For this review, use the dimensioned drawing (mm, ordinates from the lowest corner) and the shaded views. Give positions to 0.01 mm unless a question says otherwise; leave off trailing zeros. Order: outer loops, then holes, each group sorted by start corner. A loop starts at its lowest first (then second) coordinate and runs counter-clockwise, first axis right, second up.
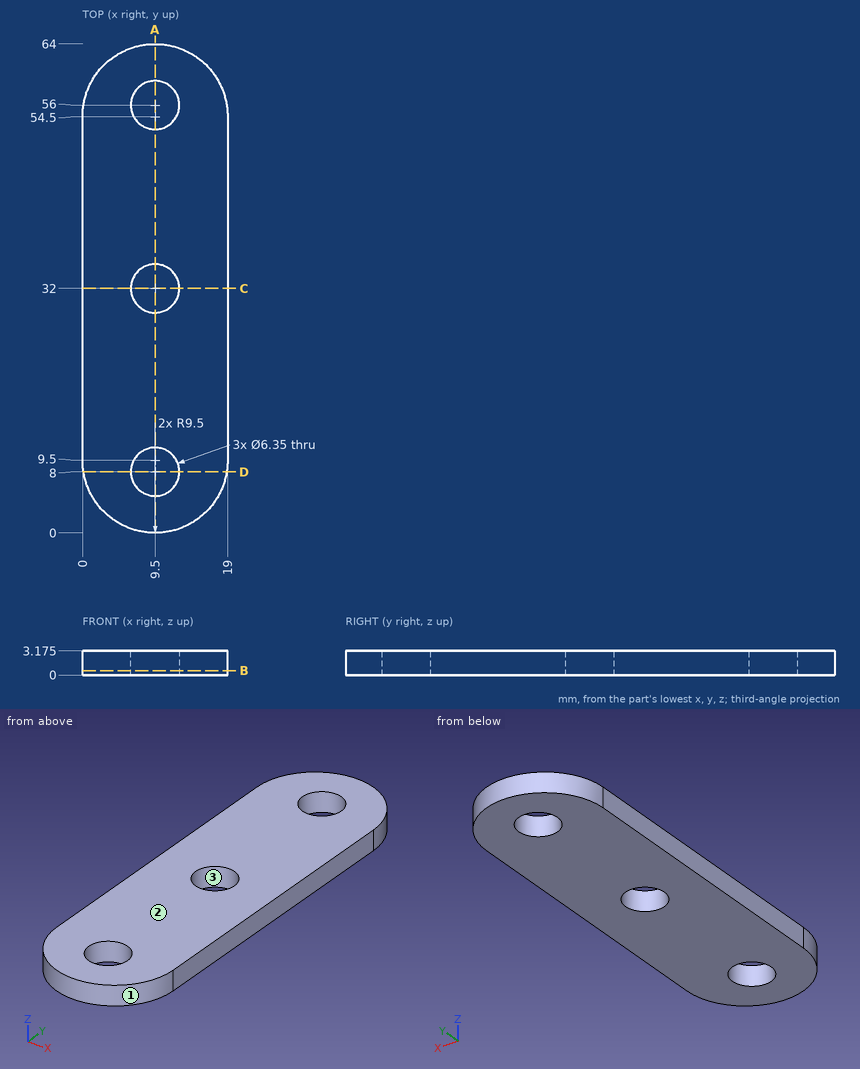
1. For pin 1 (5 mm diameter, centred on x = 9.5, y = 8, fed in from +Z), flat-tipped, find the tip position at first contact; note if it passes through.
Recorded:
pin 1: passes through
2. Draft analysis for pull direction X (two halves, no side actions). For the marked faces 1, 2 and 3, state which applies: pulls with the +X half, pulls with the -X half, needs draft (parallel to the pull), parting line crosses it, or undercut.
Recorded:
face 1: parting line crosses it
face 2: needs draft
face 3: undercut
3. For line 1 along Y through (x, z) = (9.5, 2) (3 decimals); line 2 along Y through (x, z) = (10.25, 2.35); line 3 along X through (y, z) = (54, 0.45), list the stretches that pass through material, from the lowest coordinate up.
Recorded:
line 1: y = 0 to 4.825, 11.175 to 28.825, 35.175 to 52.825, 59.175 to 64
line 2: y = 0.03 to 4.91, 11.09 to 28.91, 35.09 to 52.91, 59.09 to 63.97
line 3: x = 0 to 7.03, 11.97 to 19
4. Take a section at D-D (y = 8). State the section outline as (x, z) points (3 decimals).
Recorded:
outline: (0.119, 0) - (6.325, 0) - (6.325, 3.175) - (0.119, 3.175) - close; (12.675, 0) - (18.881, 0) - (18.881, 3.175) - (12.675, 3.175) - close
5. Take a section at A-A (x = 9.5). State the section outline as (y, z) points (3 decimals), then the cut area to 3 significant figures.
Recorded:
outline: (0, 0) - (4.825, 0) - (4.825, 3.175) - (0, 3.175) - close; (11.175, 0) - (28.825, 0) - (28.825, 3.175) - (11.175, 3.175) - close; (35.175, 0) - (52.825, 0) - (52.825, 3.175) - (35.175, 3.175) - close; (59.175, 0) - (64, 0) - (64, 3.175) - (59.175, 3.175) - close
area: 143 mm2
6. Take a section at B-B (z = 0.6). State the section outline as (x, y) points (3 decimals), then the cut area to 3 significant figures.
Recorded:
outline: (0, 9.5) arc R9.5 ccw to (19, 9.5) - (19, 54.5) arc R9.5 ccw to (0, 54.5) - close; hole circle Ø6.35 at (9.5, 8); hole circle Ø6.35 at (9.5, 32); hole circle Ø6.35 at (9.5, 56)
area: 1,040 mm2
7. Take a section at C-C (y = 32). State the section outline as (x, z) points (3 decimals), then the cut area to 3 significant figures.
Recorded:
outline: (0, 0) - (6.325, 0) - (6.325, 3.175) - (0, 3.175) - close; (12.675, 0) - (19, 0) - (19, 3.175) - (12.675, 3.175) - close
area: 40.2 mm2
